Answer from the drawing. Dimensions are ordinates in mm from the lowest x, y and z of the part. Round coordinates to 2 decimals unless told otherwise and drop trailing zeros. Loops run counter-clockwise (first coordinate to the right, second up) from the corner with the lowest first, then second, coordinate; pieces in that order, holes last. Notation, with made-up numbers: M -26.5,-35 L 6.5,-35 A21 cw 6.5,4 Z; hole C 34.5,44 d7. An arc over 180 degrees is marked long. Answer as CSV lines item,"result".
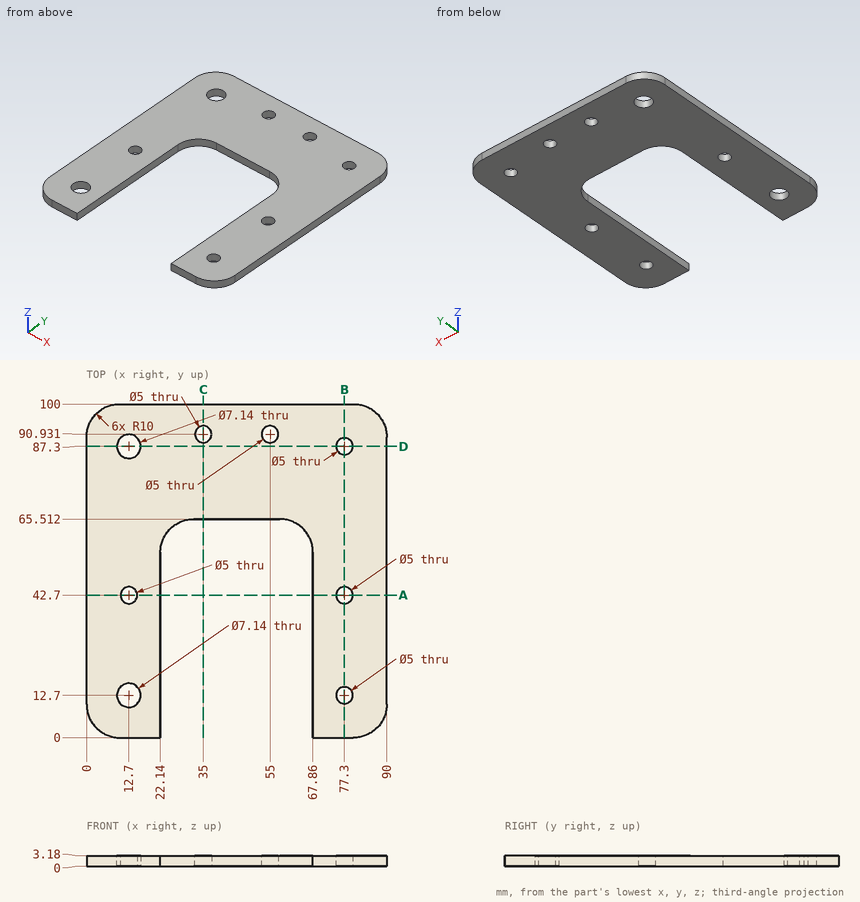
1) Find section D-D, the plane y = 87.3. Give the vertices of the cut face in (x, z), then the cut area to 3 significant figures.
Evaluation:
outline,"M 0,0 L 9.13,0 L 9.13,3.18 L 0,3.18 Z; M 16.27,0 L 74.8,0 L 74.8,3.18 L 16.27,3.18 Z; M 79.8,0 L 90,0 L 90,3.18 L 79.8,3.18 Z"
area,"248 mm^2"
2) Find section A-A, the plane y = 42.7. Give the vertices of the cut face in (x, z).
Evaluation:
outline,"M 0,0 L 10.2,0 L 10.2,3.18 L 0,3.18 Z; M 15.2,0 L 22.14,0 L 22.14,3.18 L 15.2,3.18 Z; M 67.86,0 L 74.8,0 L 74.8,3.18 L 67.86,3.18 Z; M 79.8,0 L 90,0 L 90,3.18 L 79.8,3.18 Z"
3) Straight lines are drawn through the part: line 1 (Y direction, x = 77.3, z = 2.3); line 2 (X direction, y = 42.7, z = 1.85); line 3 (X direction, y = 28.5, z = 0.6). For each, find the intervals that lie inside material, in ascending order.
Evaluation:
line 1,"y = 0 to 10.2, 15.2 to 40.2, 45.2 to 84.8, 89.8 to 100"
line 2,"x = 0 to 10.2, 15.2 to 22.14, 67.86 to 74.8, 79.8 to 90"
line 3,"x = 0 to 22.14, 67.86 to 90"
4) Each of these flat-tipped pins is pushed along its axis until it touches: P1, Ø1, axis at x = 49.5, z = 1, coming from the -Y side; P2, Ø4, axis at x = 35, y = 90.93, coming from the -Z side. Where does it stop, or does it pass through?
Evaluation:
P1,"stops at y = 65.51"
P2,"passes through"
5) Find section B-B, the plane x = 77.3. Give the vertices of the cut face in (y, z).
Evaluation:
outline,"M 0,0 L 10.2,0 L 10.2,3.18 L 0,3.18 Z; M 15.2,0 L 40.2,0 L 40.2,3.18 L 15.2,3.18 Z; M 45.2,0 L 84.8,0 L 84.8,3.18 L 45.2,3.18 Z; M 89.8,0 L 100,0 L 100,3.18 L 89.8,3.18 Z"
6) Find section C-C, the plane x = 35. Give the vertices of the cut face in (y, z).
Evaluation:
outline,"M 65.51,0 L 88.43,0 L 88.43,3.18 L 65.51,3.18 Z; M 93.43,0 L 100,0 L 100,3.18 L 93.43,3.18 Z"
